Autodesk Inventor part; units mm, degrees
ref_plane "YZ Plane" through (0, 0, 0) normal (1, 0, 0) x (0, 1, 0)
ref_plane "XZ Plane" through (0, 0, 0) normal (0, 1, 0) x (-1, 0, 0)
ref_plane "XY Plane" through (0, 0, 0) normal (0, 0, 1) x (1, 0, 0)
sketch "Sketch1" plane through (0, 0, 0) normal (0, 1, 0) x (-1, 0, 0)
  line L0 (0, 0) -> (50.8, 0)
  line L1 (50.8, 0) -> (50.8, -660.4)
  line L2 (50.8, -660.4) -> (0, -660.4)
  line L3 (0, -660.4) -> (0, 0)
  dimension "d0" = 50.8
  dimension "d1" = 660.4
extrude "Extrusion1" add sketch "Sketch1" along normal blind 25.4
sketch "Sketch3" plane through (-50.8, 0, 0) normal (0, 0, 1) x (1, 0, 0)
  line L0 (3.175, 22.225) -> (47.625, 22.225)
  line L1 (47.625, 22.225) -> (47.625, 3.175)
  line L2 (47.625, 3.175) -> (3.175, 3.175)
  line L3 (3.175, 3.175) -> (3.175, 22.225)
  line L4 (0, 25.4) -> (50.8, 25.4)
  line L5 (0, 0) -> (0, 25.4)
  line L6 (50.8, 0) -> (0, 0)
  line L7 (50.8, 0) -> (50.8, 25.4)
  dimension "d16" = 3.175
  dimension "d17" = 3.175
  dimension "d18" = 3.175
  dimension "d19" = 3.175
extrude "Extrusion3" cut sketch "Sketch3" against normal blind 660.4 contours L0 L1 L2 L3
sketch "Sketch4" plane through (0, 0, 0) normal (1, 0, 0) x (0, 0, -1)
  circle A0 centre (12.7, 12.7) radius 1.9685
  line L0 (0, 25.4) -> (660.4, 25.4)
  line L1 (0, 0) -> (0, 25.4)
  circle A1 centre (38.1, 12.7) radius 1.9685
  circle A2 centre (63.5, 12.7) radius 1.9685
  circle A3 centre (88.9, 12.7) radius 1.9685
  circle A4 centre (114.3, 12.7) radius 1.9685
  circle A5 centre (139.7, 12.7) radius 1.9685
  circle A6 centre (165.1, 12.7) radius 1.9685
  circle A7 centre (190.5, 12.7) radius 1.9685
  circle A8 centre (215.9, 12.7) radius 1.9685
  circle A9 centre (241.3, 12.7) radius 1.9685
  circle A10 centre (266.7, 12.7) radius 1.9685
  circle A11 centre (292.1, 12.7) radius 1.9685
  circle A12 centre (317.5, 12.7) radius 1.9685
  circle A13 centre (342.9, 12.7) radius 1.9685
  circle A14 centre (368.3, 12.7) radius 1.9685
  circle A15 centre (393.7, 12.7) radius 1.9685
  circle A16 centre (419.1, 12.7) radius 1.9685
  circle A17 centre (444.5, 12.7) radius 1.9685
  circle A18 centre (469.9, 12.7) radius 1.9685
  circle A19 centre (495.3, 12.7) radius 1.9685
  circle A20 centre (520.7, 12.7) radius 1.9685
  circle A21 centre (546.1, 12.7) radius 1.9685
  circle A22 centre (571.5, 12.7) radius 1.9685
  circle A23 centre (596.9, 12.7) radius 1.9685
  circle A24 centre (622.3, 12.7) radius 1.9685
  circle A25 centre (647.7, 12.7) radius 1.9685
  dimension "d22" = 3.937
  dimension "d23" = 12.7
  dimension "d24" = 12.7
  dimension "d27" = 25.4
extrude "Extrusion4" cut sketch "Sketch4" against normal blind 50.8
sketch "Sketch5" plane through (0, 25.4, 0) normal (0, 1, 0) x (1, 0, 0)
  circle A0 centre (-25.4, 355.6) radius 11.43
  line L0 (-50.8, 660.4) -> (-50.8, 0)
  circle A1 centre (-25.4, 647.7) radius 2.54
  line L1 (0, 660.4) -> (-50.8, 660.4)
  point P0 (0, 0)
  dimension "d34" = 22.86
  dimension "d35" = 25.4
  dimension "d36" = 304.8
  dimension "d39" = 5.08
  dimension "d40" = 25.4
  dimension "d41" = 12.7
extrude "Extrusion5" cut sketch "Sketch5" against normal blind 25.4
properties part number "kermit frame 8"
Here's how the part is built. I have some questions about the finished solid (model axes, mm). A direction names the side the tool comes from. Round coordinates to 2 decimals unless told otherwise and drop trailing zeros. Loops run counter-clockwise (first coordinate to the right, second up) from the corner with the lowest first, then second, coordinate; pieces in that order, holes last.
1. Thinking about a two-plate mould opening in Y: for faces 3 (the face through (-25, 25.4, -326)), 4 (the face through (-50.8, 13, -326)), 5 (the face through (-26, 22.225, -326)), 6 (the face through (-47.625, 13, -326)), which applies, released by +Y, released by -Y, zero draft, split by the parting line, or undercut?
Answers:
face 3: released by +Y
face 4: zero draft
face 5: undercut
face 6: undercut
2. If I drill on probe 1 along X at (y, z) = (23.4, -647.7); probe 2 along Y at (x, z) = (-49.55, -368.3); probe 3 along X at (y, z) = (10.25, -315) (3 decimals), over which ranges is the centre line in solid material (lowest first)?
Answers:
probe 1: x = -50.8 to -27.94, -22.86 to 0
probe 2: y = 0 to 10.73, 14.67 to 25.4
probe 3: x = -50.8 to -47.625, -3.175 to 0
3. Suppose I cut it at A-A, the plane z = -355.6. Please give me the cut outline in (x, y) (3 decimals), and give its area (3 significant figures).
Answers:
outline: (-50.8, 0) - (-36.83, 0) - (-36.83, 3.175) - (-47.625, 3.175) - (-47.625, 22.225) - (-36.83, 22.225) - (-36.83, 25.4) - (-50.8, 25.4) - close; (-13.97, 0) - (0, 0) - (0, 25.4) - (-13.97, 25.4) - (-13.97, 22.225) - (-3.175, 22.225) - (-3.175, 3.175) - (-13.97, 3.175) - close
area: 298 mm2
4. For faces 1 (the face through (-25, 3.175, -326)), 2 (the face through (0, 13, -335)), which set-ups out of +Z, -Z, +X, -X, +Y, -Y let a thin tool reach every point of the face, with its end or its side?
Answers:
face 1: +Z, -Z
face 2: +Z, -Z, +X, +Y, -Y
